```python
from build123d import *

# Parameters (mm, degrees)
PAD007_DEPTH    = 10
SKETCH016_R     = 1.5
SKETCH016_W     = 80
SKETCH016_H     = 10.5
POCKET008_DEPTH = 7
SKETCH017_W     = 9.5
SKETCH017_H     = 9.5
POCKET009_DEPTH = 2
SKETCH018_W     = 6
SKETCH018_H     = 6
POCKET010_DEPTH = 5
SKETCH019_R     = 1.5
POCKET011_DEPTH = 6
SKETCH020_R     = 1.5
POCKET012_DEPTH = 6


with BuildPart() as part:
    # Sketch015 → Pad007 (new body)
    with BuildSketch(Plane.XY):
        Polygon((45.5, 7.5), (45.5, -7.5), (37.5, -7.5), (37.5, -15.5), (29.5, -15.5), (29.5, -7.5), (-45.5, -7.5), (-45.5, 7.5), (-37.5, 7.5), (-37.5, 15.5), (-29.5, 15.5), (-29.5, 7.5), align=None)
    extrude(amount=PAD007_DEPTH)

    # Sketch016 (on Face14 of Pad007) → Pocket008 (cut)
    with BuildSketch(Plane.XY.offset(10)):
        with Locations((-33.5, 11.5)):
            Circle(SKETCH016_R)
        with Locations((33.5, -11.5)):
            Circle(SKETCH016_R)
        Rectangle(SKETCH016_W, SKETCH016_H)
    extrude(amount=-POCKET008_DEPTH, mode=Mode.SUBTRACT)

    # Sketch017 (on Face23 of Pocket008) → Pocket009 (cut)
    with BuildSketch(Plane.XY.offset(3)):
        Rectangle(SKETCH017_W, SKETCH017_H)
    extrude(amount=-POCKET009_DEPTH, mode=Mode.SUBTRACT)

    # Sketch018 (on Face28 of Pocket009) → Pocket010 (cut)
    with BuildSketch(Plane.XY.offset(1)):
        Rectangle(SKETCH018_W, SKETCH018_H)
    extrude(amount=-POCKET010_DEPTH, mode=Mode.SUBTRACT)

    # Sketch019 (on Face1 of Pocket010) → Pocket011 (cut)
    with BuildSketch(Plane.YZ.offset(45.5)):
        with Locations((0, 5)):
            Circle(SKETCH019_R)
    extrude(amount=-POCKET011_DEPTH, mode=Mode.SUBTRACT)

    # Sketch020 (on Face15 of Pocket011) → Pocket012 (cut)
    with BuildSketch(Plane(origin=(-45.5, 0, 0), x_dir=(0, -1, 0), z_dir=(-1, 0, 0))):
        with Locations((0, 5)):
            Circle(SKETCH020_R)
    extrude(amount=-POCKET012_DEPTH, mode=Mode.SUBTRACT)


solid = part.part
```
Model file for the job. Use its own axes, mm. A direction names the side the tool comes from. Coordinates: 2 decimals unless noted, no trailing zeros. Order: outer loops, then holes, each group sorted by start corner. A loop starts at its lowest first (then second) coordinate and runs counter-clockwise, first axis right, second up. Notation, with made-up numbers: M 2,3.25 L 59,3.25 A5 ccw 59,7.25 Z; hole C 2,13 d11. An arc over 180 degrees is marked long. Answer as CSV lines item,"result".
(1) Band-saw the part on B-B, the plane y = 0. List the corners of the cut face in (x, z), then the cut area to 3 significant figures.
Geometry says:
outline,"M -45.5,0 L -3,0 L -3,1 L -4.75,1 L -4.75,3 L -40,3 L -40,3.5 L -45.5,3.5 Z; M -45.5,6.5 L -40,6.5 L -40,10 L -45.5,10 Z; M 3,0 L 45.5,0 L 45.5,3.5 L 40,3.5 L 40,3 L 4.75,3 L 4.75,1 L 3,1 Z; M 40,6.5 L 45.5,6.5 L 45.5,10 L 40,10 Z"
area,"292 mm2"
(2) Band-saw the part on D-D, the plane y = -11.5. List the corners of the cut face in (x, z), then the cut area to 3 significant figures.
Geometry says:
outline,"M 29.5,0 L 37.5,0 L 37.5,10 L 35,10 L 35,3 L 32,3 L 32,10 L 29.5,10 Z"
area,"59.0 mm2"
(3) Flat gauge pins, fed straight in: pin 1 (5 mm diameter, centred on x = -1.5, y = 1.5, fed in from +Z); pin 2 (1.5 mm diameter, centred on x = 3, z = 2, fed in from -Y); pin 3 (5 mm diameter, centred on x = 14, z = 4.5, fed in from +Y). Where does each tip first touch, or does it go through?
Geometry says:
pin 1,"stops at z = 1"
pin 2,"stops at y = -7.5"
pin 3,"stops at y = 7.5"
(4) Wall check: line 1 along Y through (x, z) = (-33.5, 8); line 2 along Y through (x, z) = (33.5, 5.5); line 3 along Z through (x, y) = (-44.15, 0). Give the ranges that are in metal, low to high.
Geometry says:
line 1,"y = -7.5 to -5.25, 5.25 to 10, 13 to 15.5"
line 2,"y = -15.5 to -13, -10 to -5.25, 5.25 to 7.5"
line 3,"z = 0 to 3.5, 6.5 to 10"
(5) 3-axis set-ups, long thin cutter, end or side, ignore diameter. For faces 1 (the flat face through (7, 7.5, 5)), 2 (the flat face through (37.5, -11, 5)), 3 (the flat face through (-7, -7.5, 5)), 4 (the flat face through (-9, 0, 3)): which of +Z, -Z, +X, -X, +Y, -Y reach the whole face in a straight line?
Geometry says:
face 1,"+Z, -Z, +X, +Y"
face 2,"+Z, -Z, +X, -Y"
face 3,"+Z, -Z, -X, -Y"
face 4,"+Z"
(6) Pull direction Y, two halves, no side cores. Call faces 5 (the flat face through (42, -7.5, 5)), 6 (the flat face through (-37.5, 11, 5)), 7 (the flat face through (-34, 12, 3)): +Y half, -Y half, draft (parallel to the pull), parting line (faces both ways), or undercut.
Geometry says:
face 5,"-Y half"
face 6,"draft"
face 7,"undercut"
(7) Band-saw the part on C-C, the plane z = 7.5. List the corners of the cut face in (x, y), then the cut area to 3 significant figures.
Geometry says:
outline,"M -45.5,-7.5 L 29.5,-7.5 L 29.5,-15.5 L 37.5,-15.5 L 37.5,-7.5 L 45.5,-7.5 L 45.5,7.5 L -29.5,7.5 L -29.5,15.5 L -37.5,15.5 L -37.5,7.5 L -45.5,7.5 Z; hole M -40,-5.25 L 40,-5.25 L 40,5.25 L -40,5.25 Z; hole C -33.5,11.5 d3; hole C 33.5,-11.5 d3"
area,"639 mm2"
(8) Band-saw the part on A-A, the plane x = 26. List the corners of the cut face in (y, z), then the cut area to 3 significant figures.
Geometry says:
outline,"M -7.5,0 L 7.5,0 L 7.5,10 L 5.25,10 L 5.25,3 L -5.25,3 L -5.25,10 L -7.5,10 Z"
area,"76.5 mm2"
